Verification items for the finished model (mm, model axes). Coordinates: 2 decimals unless noted, no trailing zeros.
Q1. Sectioned sample at A-A (z = 1.6). Count the separate pieces of the cut face and the enclosed holes in it, then the cut area to 3 significant figures.
Q2. Go/stop test with flat-tipped pins: P1, Ø1.2, axis at x = 0.5, z = 2, coming from the -Y side; P2, Ø1.2, axis at y = -124.5, z = 1.5, coming from the -X side; P3, Ø1.2, axis at x = 2, z = 1.5, coming from the +Y side; P4, Ø3, axis at x = -100, y = 62.735, coming from the +Z side. Record where each tip stops, or that it passes through.
Q3. Material ranges on probe 1 along Y at (x, z) = (-73, 0.9); probe 2 along Y at (x, z) = (26.1, 0.9); probe 3 along X at (y, z) = (-28, 0.95), recorded low to high.
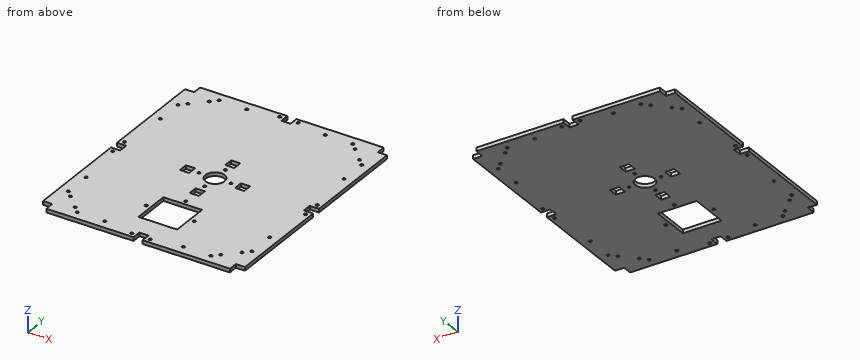
```python
from build123d import *

# Parameters (mm, degrees)
F0_R     = 1.55
F0_W     = 42.2
F0_H     = 42.2
F0_W_2   = 10
F0_H_2   = 10
F0_R_2   = 10.5
F1_DEPTH = 4


with BuildPart() as f1:
    # F0 (on Top) → F1 (new body)
    with BuildSketch(Plane.XY):
        Polygon((-100, 120), (-110, 120), (-110, 5), (-100, 5), (-100, -5), (-110, -5), (-110, -120), (-100, -120), (-100, -130), (-5, -130), (-5, -120), (5, -120), (5, -130), (100, -130), (100, -120), (110, -120), (110, -5), (100, -5), (100, 5), (110, 5), (110, 120), (100, 120), (100, 130), (5, 130), (5, 120), (-5, 120), (-5, 130), (-100, 130), align=None)
        with Locations((-93.438403, -99.296597)):
            Circle(F0_R, mode=Mode.SUBTRACT)
        with Locations((-72.735, -120)):
            Circle(F0_R, mode=Mode.SUBTRACT)
        with Locations((-79.296597, -113.438403)):
            Circle(F0_R, mode=Mode.SUBTRACT)
        with Locations((-100, -92.735)):
            Circle(F0_R, mode=Mode.SUBTRACT)
        with Locations((-42.735, -120)):
            Circle(F0_R, mode=Mode.SUBTRACT)
        with Locations((-10, -125)):
            Circle(F0_R, mode=Mode.SUBTRACT)
        with Locations((-26.1, -75.647)):
            Circle(F0_R, mode=Mode.SUBTRACT)
        with Locations((-100, -62.735)):
            Circle(F0_R, mode=Mode.SUBTRACT)
        with Locations((-105, -10)):
            Circle(F0_R, mode=Mode.SUBTRACT)
        with Locations((10, -125)):
            Circle(F0_R, mode=Mode.SUBTRACT)
        with Locations((42.735, -120)):
            Circle(F0_R, mode=Mode.SUBTRACT)
        with Locations((0, -75.647)):
            Rectangle(F0_W, F0_H, mode=Mode.SUBTRACT)
        with Locations((26.1, -75.647)):
            Circle(F0_R, mode=Mode.SUBTRACT)
        with Locations((72.735, -120)):
            Circle(F0_R, mode=Mode.SUBTRACT)
        with Locations((79.296597, -113.438403)):
            Circle(F0_R, mode=Mode.SUBTRACT)
        with Locations((93.438403, -99.296597)):
            Circle(F0_R, mode=Mode.SUBTRACT)
        with Locations((100, -92.735)):
            Circle(F0_R, mode=Mode.SUBTRACT)
        with Locations((0, -49.547)):
            Circle(F0_R, mode=Mode.SUBTRACT)
        with Locations((0, -30)):
            Rectangle(F0_W_2, F0_H_2, mode=Mode.SUBTRACT)
        with Locations((0, -17.5)):
            Circle(F0_R, mode=Mode.SUBTRACT)
        with Locations((100, -62.735)):
            Circle(F0_R, mode=Mode.SUBTRACT)
        with Locations((105, -10)):
            Circle(F0_R, mode=Mode.SUBTRACT)
        with Locations((-105, 10)):
            Circle(F0_R, mode=Mode.SUBTRACT)
        with Locations((-100, 62.735)):
            Circle(F0_R, mode=Mode.SUBTRACT)
        with Locations((-30, 0)):
            Rectangle(F0_W_2, F0_H_2, mode=Mode.SUBTRACT)
        with Locations((-17.5, 0)):
            Circle(F0_R, mode=Mode.SUBTRACT)
        with Locations((-100, 92.735)):
            Circle(F0_R, mode=Mode.SUBTRACT)
        with Locations((-93.438403, 99.296597)):
            Circle(F0_R, mode=Mode.SUBTRACT)
        with Locations((-79.296597, 113.438403)):
            Circle(F0_R, mode=Mode.SUBTRACT)
        with Locations((-72.735, 120)):
            Circle(F0_R, mode=Mode.SUBTRACT)
        with Locations((-42.735, 120)):
            Circle(F0_R, mode=Mode.SUBTRACT)
        with Locations((-10, 125)):
            Circle(F0_R, mode=Mode.SUBTRACT)
        Circle(F0_R_2, mode=Mode.SUBTRACT)
        with Locations((17.5, 0)):
            Circle(F0_R, mode=Mode.SUBTRACT)
        with Locations((0, 17.5)):
            Circle(F0_R, mode=Mode.SUBTRACT)
        with Locations((0, 30)):
            Rectangle(F0_W_2, F0_H_2, mode=Mode.SUBTRACT)
        with Locations((30, 0)):
            Rectangle(F0_W_2, F0_H_2, mode=Mode.SUBTRACT)
        with Locations((105, 10)):
            Circle(F0_R, mode=Mode.SUBTRACT)
        with Locations((100, 62.735)):
            Circle(F0_R, mode=Mode.SUBTRACT)
        with Locations((10, 125)):
            Circle(F0_R, mode=Mode.SUBTRACT)
        with Locations((42.735, 120)):
            Circle(F0_R, mode=Mode.SUBTRACT)
        with Locations((100, 92.735)):
            Circle(F0_R, mode=Mode.SUBTRACT)
        with Locations((79.296597, 113.438403)):
            Circle(F0_R, mode=Mode.SUBTRACT)
        with Locations((72.735, 120)):
            Circle(F0_R, mode=Mode.SUBTRACT)
        with Locations((93.438403, 99.296597)):
            Circle(F0_R, mode=Mode.SUBTRACT)
    extrude(amount=F1_DEPTH)


solid = f1.part
```
Geometry check:
1. separate pieces: 1
1. enclosed holes: 45
1. area: 53,600 mm2
2. P1: stops at y = -120
2. P2: stops at x = -100
2. P3: stops at y = 120
2. P4: passes through
3. probe 1: y = -130 to -121.53, -118.47 to 118.47, 121.53 to 130
3. probe 2: y = -130 to -77.2, -74.1 to -5, 5 to 130
3. probe 3: x = -110 to -5, 5 to 110
